from build123d import *

# Parameters (mm, degrees)
F0_R      = 12.45
F1_DEPTH  = 12
F2_R      = 14.5
F3_DEPTH  = 3
F4_R      = 9.95
F5_DEPTH  = 70
F7_DEPTH  = 20
F10_DEPTH = 10
F11_SIZE  = 1
F12_R     = 0.5


with BuildPart() as f1:
    # F0 (on Front) → F1 (new body)
    with BuildSketch(Plane.XZ):
        Circle(F0_R)
    extrude(amount=-F1_DEPTH)

    # F2 (on Front) → F3 (join)
    with BuildSketch(Plane.XZ):
        Circle(F2_R)
    extrude(amount=F3_DEPTH)

    # F4 (on face) → F5 (join)
    with BuildSketch(Plane.XZ.offset(3)):
        Circle(F4_R)
    extrude(amount=F5_DEPTH)

    # F6 (on face) → F7 (join)
    with BuildSketch(Plane.XZ.offset(3)):
        with BuildLine():
            Line((2, 9.7469225913), (2, 12.3389626793))
            ThreePointArc((2, 12.3389626793), (0, 12.5), (-2, 12.3389626793))
            Line((-2, 12.3389626793), (-2, 9.7469225913))
            ThreePointArc((-2, 9.7469225913), (0, 9.95), (2, 9.7469225913))
        make_face()
        with BuildLine():
            ThreePointArc((-7.3471313431, 6.7098555146), (-5.8484632603, 8.049719094), (-4.1110633656, 9.0609965238))
            Line((-4.1110633656, 9.0609965238), (-5.6346263027, 11.1580010051))
            ThreePointArc((-5.6346263027, 11.1580010051), (-7.3473156537, 10.1127124297), (-8.8706942802, 8.8068599959))
            Line((-8.8706942802, 8.8068599959), (-7.3471313431, 6.7098555146))
        make_face()
        with BuildLine():
            ThreePointArc((-9.887908233, 1.109851691), (-9.4630123371, 3.074719094), (-8.6518402555, 4.9140777561))
            Line((-8.6518402555, 4.9140777561), (-11.1170168717, 5.7150621934))
            ThreePointArc((-11.1170168717, 5.7150621934), (-11.8882064537, 3.8627124297), (-12.3530848492, 1.9108361283))
            Line((-12.3530848492, 1.9108361283), (-9.887908233, 1.109851691))
        make_face()
        with BuildLine():
            ThreePointArc((-8.6518402555, -4.9140777561), (-9.4630123371, -3.074719094), (-9.887908233, -1.109851691))
            Line((-9.887908233, -1.109851691), (-12.3530848492, -1.9108361283))
            ThreePointArc((-12.3530848492, -1.9108361283), (-11.8882064537, -3.8627124297), (-11.1170168717, -5.7150621934))
            Line((-11.1170168717, -5.7150621934), (-8.6518402555, -4.9140777561))
        make_face()
        with BuildLine():
            ThreePointArc((-4.1110633656, -9.0609965238), (-5.8484632603, -8.049719094), (-7.3471313431, -6.7098555146))
            Line((-7.3471313431, -6.7098555146), (-8.8706942802, -8.8068599959))
            ThreePointArc((-8.8706942802, -8.8068599959), (-7.3473156537, -10.1127124297), (-5.6346263027, -11.1580010051))
            Line((-5.6346263027, -11.1580010051), (-4.1110633656, -9.0609965238))
        make_face()
        with BuildLine():
            ThreePointArc((2, -9.7469225913), (0, -9.95), (-2, -9.7469225913))
            Line((-2, -9.7469225913), (-2, -12.3389626793))
            ThreePointArc((-2, -12.3389626793), (0, -12.5), (2, -12.3389626793))
            Line((2, -12.3389626793), (2, -9.7469225913))
        make_face()
        with BuildLine():
            Line((8.8706942802, -8.8068599959), (7.3471313431, -6.7098555146))
            ThreePointArc((7.3471313431, -6.7098555146), (5.8484632603, -8.049719094), (4.1110633656, -9.0609965238))
            Line((4.1110633656, -9.0609965238), (5.6346263027, -11.1580010051))
            ThreePointArc((5.6346263027, -11.1580010051), (7.3473156537, -10.1127124297), (8.8706942802, -8.8068599959))
        make_face()
        with BuildLine():
            Line((12.3530848492, -1.9108361283), (9.887908233, -1.109851691))
            ThreePointArc((9.887908233, -1.109851691), (9.4630123371, -3.074719094), (8.6518402555, -4.9140777561))
            Line((8.6518402555, -4.9140777561), (11.1170168717, -5.7150621934))
            ThreePointArc((11.1170168717, -5.7150621934), (11.8882064537, -3.8627124297), (12.3530848492, -1.9108361283))
        make_face()
        with BuildLine():
            Line((11.1170168717, 5.7150621934), (8.6518402555, 4.9140777561))
            ThreePointArc((8.6518402555, 4.9140777561), (9.4630123371, 3.074719094), (9.887908233, 1.109851691))
            Line((9.887908233, 1.109851691), (12.3530848492, 1.9108361283))
            ThreePointArc((12.3530848492, 1.9108361283), (11.8882064537, 3.8627124297), (11.1170168717, 5.7150621934))
        make_face()
        with BuildLine():
            Line((5.6346263027, 11.1580010051), (4.1110633656, 9.0609965238))
            ThreePointArc((4.1110633656, 9.0609965238), (5.8484632603, 8.049719094), (7.3471313431, 6.7098555146))
            Line((7.3471313431, 6.7098555146), (8.8706942802, 8.8068599959))
            ThreePointArc((8.8706942802, 8.8068599959), (7.3473156537, 10.1127124297), (5.6346263027, 11.1580010051))
        make_face()
    extrude(amount=F7_DEPTH)

    # F9 (on offset) → F10 (cut)
    with BuildSketch(Plane.XY.offset(6)):
        with BuildLine():
            Line((-3, -55), (-3, -85))
            Line((-3, -85), (3, -85))
            Line((3, -85), (3, -55))
            ThreePointArc((3, -55), (0, -52), (-3, -55))
        make_face()
    extrude(amount=F10_DEPTH, mode=Mode.SUBTRACT)

    # F11
    f11_edges = [f1.edges().sort_by_distance(p)[0] for p in [
        (-5.880157, -73, -8.026596),
    ]]
    chamfer(f11_edges, length=F11_SIZE)

    # F12
    f12_edges = [f1.edges().sort_by_distance(p)[0] for p in [
        (-3, -63.5, 9.486965),
        (0, -52, 9.95),
        (3, -63.5, 9.486965),
    ]]
    fillet(f12_edges, radius=F12_R)


solid = f1.part
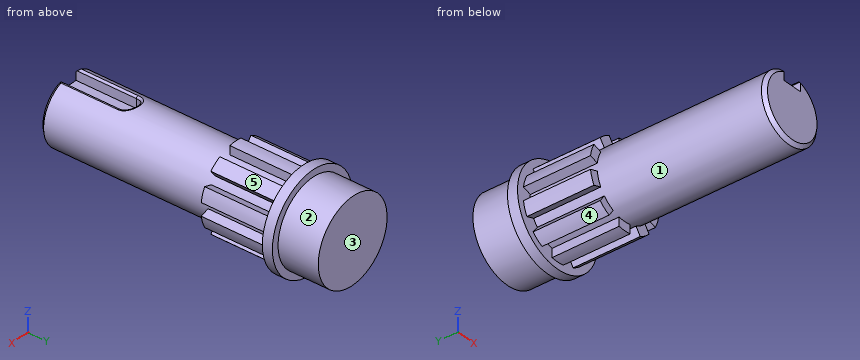
The model under review builds one solid part; all positions refer to its coordinate system, in mm. Face numbers are marked on the shaded views. A direction names the side the tool comes from. Round coordinates to 2 decimals unless told otherwise and drop trailing zeros. Loops run counter-clockwise (first coordinate to the right, second up) from the corner with the lowest first, then second, coordinate; pieces in that order, holes last. Notation, with made-up numbers: (72.25, 32.25) - (126.25, 32.25) arc R36 ccw to (126.25, 71.25) - close; hole circle Ø10 at (89, 42.25). An arc over 180 degrees is marked (long way). Use CSV: the item, a comma, the result in double quotes.
(1) For line 1 (X direction, y = -30, z = 0.25); line 2 (Z direction, x = -0.5, y = -55); line 3 (Y direction, x = -10, z = -3.25), list the stretches that pass through material, from the lowest coordinate up.
Working result:
line 1,"x = -9.95 to 9.95"
line 2,"z = -9.94 to 6"
line 3,"y = -23 to 12"
(2) Take a section at B-B, the plane y = 7.5. Give the boundary of the cut face in (x, z), plus the area to 3 significant figures.
Working result:
outline,"circle Ø24.9 at (0, 0)"
area,"487 mm^2"
(3) Clearance check with flat-ended pins moving along their axes: P1, Ø0.8, axis at y = -12.5, z = -11.5, coming from the -X side; P2, Ø2, axis at x = 0.5, z = -11, coming from the -Y side; P3, Ø3, axis at y = -33.5, z = -2, coming from the -X side; P4, Ø4, axis at x = -10.5, z = 2.5, coming from the -Y side. State where each tip first meets the part, or that it passes through.
Working result:
P1,"stops at x = -5.75"
P2,"stops at y = -23"
P3,"stops at x = -9.94"
P4,"stops at y = -73"
(4) Machinability: for the marked faces 1, 2, 3, 4 and 5, which of the approach directions +Z, -Z, +X, -X, +Y, -Y give a long, thin tool a straight path to every point of the face, cutting with its end or side? Answer none if there is none.
Working result:
face 1,"-Y"
face 2,"+Y"
face 3,"+Z, -Z, +X, -X, +Y"
face 4,"-Z, -X, -Y"
face 5,"+Z, +X, -Y"
(5) Take a section at A-A, the plane y = -39. Give the boundary of the cut face in (x, z).
Working result:
outline,"circle Ø19.9 at (0, 0)"
